Can you work these out from the model? Positions are in its coordinate system, mm. A direction names the side the tool comes from. Round coordinates to 2 decimals unless told otherwise and drop trailing zeros. Loops run counter-clockwise (first coordinate to the right, second up) from the corner with the lowest first, then second, coordinate; pieces in that order, holes last. Notation, with made-up numbers: M 6,52 L 61,52 A28 ccw 61,76 Z; hole C -9.5,2.25 d11. An arc over 180 degrees is marked long. Answer as CSV lines item,"result".
from build123d import *

# Parameters (mm, degrees)
F0_W     = 30
F0_H     = 30
F0_R     = 1.65
F0_R_2   = 3
F0_R_3   = 2
F0_R_4   = 1.5
F1_DEPTH = 10
F2_DEPTH = 12
F3_SIZE  = 1.5
F4_DEPTH = 4
F5_DEPTH = 8
F6_R     = 2
F7_DEPTH = 8
F6_R_2   = 1.5
F8_DEPTH = 1


# Not quite as in the source:
# - a feature names something its author has since deleted; it is built from what else it names


with BuildPart() as f1:
    # F0 (on Top) → F1 (new body)
    with BuildSketch(Plane.XY):
        with Locations((15, -15)):
            Rectangle(F0_W, F0_H)
        with Locations((9.5, -25)):
            Circle(F0_R, mode=Mode.SUBTRACT)
        with Locations((15, -24)):
            Circle(F0_R_2, mode=Mode.SUBTRACT)
        with Locations((6, -15)):
            Circle(F0_R_2, mode=Mode.SUBTRACT)
        with Locations((9.5, -5)):
            Circle(F0_R, mode=Mode.SUBTRACT)
        with Locations((15, -15)):
            Circle(F0_R_3, mode=Mode.SUBTRACT)
        with Locations((24, -15)):
            Circle(F0_R_2, mode=Mode.SUBTRACT)
        with Locations((15, -6)):
            Circle(F0_R_2, mode=Mode.SUBTRACT)
        with Locations((15, -15)):
            Circle(F0_R_3)
        with Locations((15, -6)):
            Circle(F0_R_2)
        with Locations((15, -6)):
            Circle(F0_R_4, mode=Mode.SUBTRACT)
        with Locations((15, -24)):
            Circle(F0_R_2)
        with Locations((15, -24)):
            Circle(F0_R_4, mode=Mode.SUBTRACT)
        with Locations((9.5, -5)):
            Circle(F0_R)
        with Locations((9.5, -25)):
            Circle(F0_R)
        with Locations((24, -15)):
            Circle(F0_R_2)
        with Locations((24, -15)):
            Circle(F0_R_4, mode=Mode.SUBTRACT)
        with Locations((6, -15)):
            Circle(F0_R_2)
        with Locations((6, -15)):
            Circle(F0_R_4, mode=Mode.SUBTRACT)
        with Locations((15, -24)):
            Circle(F0_R_4)
        with Locations((15, -6)):
            Circle(F0_R_4)
    extrude(amount=-F1_DEPTH)

    # F0 (on Top) → F2 (cut)
    with BuildSketch(Plane.XY):
        with Locations((15, -15)):
            Circle(F0_R_3)
    extrude(amount=-F2_DEPTH, mode=Mode.SUBTRACT)

    # F3
    f3_edges = [f1.edges().sort_by_distance(p)[0] for p in [
        (30, -30, -5),
        (0, -30, -5),
        (0, 0, -5),
        (30, 0, -5),
    ]]
    chamfer(f3_edges, length=F3_SIZE)

    # F0 (on Top) → F4 (cut)
    with BuildSketch(Plane.XY):
        with Locations((6, -15)):
            Circle(F0_R_2)
        with Locations((6, -15)):
            Circle(F0_R_4, mode=Mode.SUBTRACT)
        with Locations((24, -15)):
            Circle(F0_R_2)
        with Locations((24, -15)):
            Circle(F0_R_4, mode=Mode.SUBTRACT)
    extrude(amount=-F4_DEPTH, mode=Mode.SUBTRACT)

    # F0 (on Top) → F5 (cut)
    with BuildSketch(Plane.XY):
        with Locations((9.5, -5)):
            Circle(F0_R)
        with Locations((9.5, -25)):
            Circle(F0_R)
    extrude(amount=-F5_DEPTH, mode=Mode.SUBTRACT)

    # F6 (on face) → F7 (cut)
    with BuildSketch(Plane(origin=(0, 0, -10), x_dir=(1, 0, 0), z_dir=(0, 0, -1))):
        with BuildLine():
            ThreePointArc((19.6, 13.0404082058), (18, 15), (19.6, 16.9595917942))
            ThreePointArc((19.6, 16.9595917942), (10, 15), (19.6, 13.0404082058))
        make_face()
        with Locations((15, 15)):
            Circle(F6_R, mode=Mode.SUBTRACT)
        with BuildLine():
            ThreePointArc((19.6, 13.0404082058), (19.8989794856, 14), (20, 15))
            ThreePointArc((20, 15), (19.8989794856, 16), (19.6, 16.9595917942))
            ThreePointArc((19.6, 16.9595917942), (18, 15), (19.6, 13.0404082058))
        make_face()
    extrude(amount=-F7_DEPTH, mode=Mode.SUBTRACT)

    # F6 (on face) → F8 (cut)
    with BuildSketch(Plane(origin=(0, 0, -10), x_dir=(1, 0, 0), z_dir=(0, 0, -1))):
        with BuildLine():
            ThreePointArc((19.6, 16.9595917942), (19.8989794856, 16), (20, 15))
            ThreePointArc((20, 15), (19.8989794856, 14), (19.6, 13.0404082058))
            ThreePointArc((19.6, 13.0404082058), (19.798982076, 13.010127694), (20, 13))
            Line((20, 13), (30, 13))
            Line((30, 13), (30, 17))
            Line((30, 17), (20, 17))
            ThreePointArc((20, 17), (19.798982076, 16.989872306), (19.6, 16.9595917942))
        make_face()
        with Locations((24, 15)):
            Circle(F6_R_2, mode=Mode.SUBTRACT)
    extrude(amount=-F8_DEPTH, mode=Mode.SUBTRACT)


solid = f1.part
Item 1: If we section it at C-C on x = 12: Write out the boundary of the cut face in (y, z).
Output:
outline,"M -30,-10 L -19,-10 L -19,-2 L -11,-2 L -11,-10 L 0,-10 L 0,0 L -30,0 Z"
Item 2: If we section it at B-B on z = -2.5: Write out the boundary of the cut face in (x, y), then the cut area to 3 significant figures.
Output:
outline,"M 0,-28.5 L 1.5,-30 L 28.5,-30 L 30,-28.5 L 30,-1.5 L 28.5,0 L 1.5,0 L 0,-1.5 Z; hole C 6,-15 d6; hole C 9.5,-25 d3.3; hole C 9.5,-5 d3.3; hole C 15,-15 d10; hole C 24,-15 d6"
area,"743 mm2"
Item 3: On a 3-axis mill with a long thin cutter (end or side, diameter ignored), from which of +Z, -Z, +X, -X, +Y, -Y can I reach the whole of each face in a straight line? I mean faces 4 (the face through (25.3, -16.3, -4)), 5 (the face through (26, -15, -9)), 6 (the face through (14.9, -12.8, -2)). Say none if no direction works.
Output:
face 4,"+Z"
face 5,"-Z, +X"
face 6,"-Z"
Item 4: If we section it at A-A on x = 24: Write out the boundary of the cut face in (y, z), then the cut area to 3 significant figures.
Output:
outline,"M -30,-10 L -17,-10 L -17,-9 L -16.5,-9 L -16.5,-4 L -18,-4 L -18,0 L -30,0 Z; M -13.5,-9 L -13,-9 L -13,-10 L 0,-10 L 0,0 L -12,0 L -12,-4 L -13.5,-4 Z"
area,"257 mm2"
Item 5: If I drill on line 1 along Y through (x, z) = (9.5, -2.25); line 2 along Y through (x, z) = (24, -6.75); line 3 along Y through (x, z) = (6, -1.95), over which ranges is the centre line in solid material (lowest first)? Write a range as from..to.
Output:
line 1,"y = -30..-26.65, -23.35..-6.65, -3.35..0"
line 2,"y = -30..-16.5, -13.5..0"
line 3,"y = -30..-18, -12..0"
Item 6: Will these pins go through, and if not, where does the flat tip stop? pin 1 (6 mm diameter, centred on x = 15, y = -15, fed in from -Z); pin 2 (1 mm diameter, centred on x = 10, y = -5.5, fed in from +Z); pin 3 (3.5 mm diameter, centred on x = 6, y = -15, fed in from +Z).
Output:
pin 1,"stops at z = -2"
pin 2,"stops at z = -8"
pin 3,"stops at z = -4"
Item 7: We'd pull the mould along X, two halves only. Please class faces 1 (the face through (0.8, -29.3, -4.9)), 2 (the face through (7.3, -16.3, -4)), 3 (the face through (30, -15, -5)): released by +X, released by -X, zero draft, split by the parting line, or undercut.
Output:
face 1,"released by -X"
face 2,"undercut"
face 3,"released by +X"
Item 8: If we section it at D-D on y = -14.5: Write out the boundary of the cut face in (x, z), then the cut area to 3 significant figures.
Output:
outline,"M 0,-10 L 4.59,-10 L 4.59,-4 L 3.04,-4 L 3.04,0 L 0,0 Z; M 7.41,-10 L 10.03,-10 L 10.03,-2 L 13.06,-2 L 13.06,0 L 8.96,0 L 8.96,-4 L 7.41,-4 Z; M 16.94,-2 L 19.97,-2 L 19.97,-9 L 22.59,-9 L 22.59,-4 L 21.04,-4 L 21.04,0 L 16.94,0 Z; M 25.41,-9 L 30,-9 L 30,0 L 26.96,0 L 26.96,-4 L 25.41,-4 Z"
area,"124 mm2"
